from build123d import *

# Parameters (mm, degrees)
F0_R      = 1.75
F1_DEPTH  = 4
F3_W      = 3
F3_H      = 79.3
F4_DEPTH  = 82
F5_DEPTH  = 2
F6_DEPTH  = 2
F7_DEPTH  = 3
F8_DEPTH  = 3
F9_R      = 2
F12_DEPTH = 80.001
F14_W     = 58
F14_H     = 79.3
F14_W_2   = 22
F14_H_2   = 11
F15_DEPTH = 4


with BuildPart() as f1:
    # F0 (on Top) → F1 (new body)
    with BuildSketch(Plane.XY):
        Polygon((71, 89.45), (19, 89.45), (-6, 89.45), (-6, 81.45), (19, 81.45), (19, 15.45), (-6, 15.45), (-6, 7.45), (19, 7.45), (71, 7.45), (96, 7.45), (96, 15.45), (71, 15.45), (71, 81.45), (96, 81.45), (96, 89.45), align=None)
        with Locations((6.5, 11.45)):
            Circle(F0_R, mode=Mode.SUBTRACT)
        with Locations((83.5, 11.45)):
            Circle(F0_R, mode=Mode.SUBTRACT)
        with Locations((6.5, 85.45)):
            Circle(F0_R, mode=Mode.SUBTRACT)
        with Locations((83.5, 85.45)):
            Circle(F0_R, mode=Mode.SUBTRACT)
    extrude(amount=F1_DEPTH)

    # F3 (on offset) → F4 (join)
    with BuildSketch(Plane.XY.offset(4)):
        with Locations((20.5, 47.1)):
            Rectangle(F3_W, F3_H)
        with Locations((69.5, 47.1)):
            Rectangle(F3_W, F3_H)
    extrude(amount=F4_DEPTH)

    # F5 (cut): a face of the model
    f5_faces = [f1.faces().sort_by_distance(p)[0] for p in [
        (22, 47.1, 45),
    ]]
    extrude(f5_faces, amount=-F5_DEPTH, mode=Mode.SUBTRACT)

    # F6 (cut): a face of the model
    f6_faces = [f1.faces().sort_by_distance(p)[0] for p in [
        (68, 47.1, 45),
    ]]
    extrude(f6_faces, amount=-F6_DEPTH, mode=Mode.SUBTRACT)

    # F7 (add): a face of the model
    f7_faces = [f1.faces().sort_by_distance(p)[0] for p in [
        (71, 47.1526704697, 43.3223480034),
    ]]
    extrude(f7_faces, amount=F7_DEPTH)

    # F8 (add): a face of the model
    f8_faces = [f1.faces().sort_by_distance(p)[0] for p in [
        (19, 47.1526704697, 43.3223480034),
    ]]
    extrude(f8_faces, amount=F8_DEPTH)

    # F9
    f9_edges = [f1.edges().sort_by_distance(p)[0] for p in [
        (96, 81.45, 2),
        (96, 89.45, 2),
        (96, 15.45, 2),
        (96, 7.45, 2),
        (-6, 7.45, 2),
        (-6, 89.45, 2),
        (-6, 81.45, 2),
        (-6, 15.45, 2),
    ]]
    fillet(f9_edges, radius=F9_R)

    # F11 (on offset) → F12 (cut, through all)
    with BuildSketch(Plane.YZ.offset(74)):
        Polygon((73.4880973649, 79.5), (20.7553358046, 79.5), (17.45, 77.2472782643), (17.45, 6.3772784262), (20.6669158031, 4), (73.4427470628, 4), (76.75, 6.2499062224), (76.75, 77.1848345202), align=None)
    extrude(amount=-F12_DEPTH, mode=Mode.SUBTRACT)

    # F14 (on offset) → F15 (join)
    with BuildSketch(Plane.XY.offset(86)):
        with Locations((45, 47.1)):
            Rectangle(F14_W, F14_H)
        with Locations((55, 32.0759117305)):
            Rectangle(F14_W_2, F14_H_2, mode=Mode.SUBTRACT)
    extrude(amount=F15_DEPTH)


solid = f1.part
The model under review builds one solid part; all positions refer to its coordinate system, in mm. A direction names the side the tool comes from. Round coordinates to 2 decimals unless told otherwise and drop trailing zeros. Loops run counter-clockwise (first coordinate to the right, second up) from the corner with the lowest first, then second, coordinate; pieces in that order, holes last. Notation, with made-up numbers: M 43,79.5 L 83,79.5 A16 cw 83,106.5 Z; hole C -21.75,49.25 d4. An arc over 180 degrees is marked long. Answer as a JSON object with one key per item and string values.
Item 1: We need section C-C, the plane x = 83.5. State the section outline as (y, z) points, and give its area (3 significant figures).
Check sheet entries:
{"outline": "M 7.45,0 L 9.7,0 L 9.7,4 L 7.45,4 Z; M 13.2,0 L 15.45,0 L 15.45,4 L 13.2,4 Z; M 81.45,0 L 83.7,0 L 83.7,4 L 81.45,4 Z; M 87.2,0 L 89.45,0 L 89.45,4 L 87.2,4 Z", "area": "36.0 mm2"}
Item 2: We need section B-B, the plane z = 59. State the section outline as (x, y) points.
Check sheet entries:
{"outline": "M 16,7.45 L 20,7.45 L 20,17.45 L 16,17.45 Z; M 16,76.75 L 20,76.75 L 20,86.75 L 16,86.75 Z; M 70,7.45 L 74,7.45 L 74,17.45 L 70,17.45 Z; M 70,76.75 L 74,76.75 L 74,86.75 L 70,86.75 Z"}
Item 3: We need section A-A, the plane y = 11.45. State the section outline as (x, z) points.
Check sheet entries:
{"outline": "M -6,0 L 4.75,0 L 4.75,4 L -6,4 Z; M 8.25,0 L 81.75,0 L 81.75,4 L 74,4 L 74,90 L 16,90 L 16,4 L 8.25,4 Z; M 85.25,0 L 96,0 L 96,4 L 85.25,4 Z; hole M 20,4 L 70,4 L 70,86 L 20,86 Z"}
Item 4: Tool access review of faces 1 (the face through (6, 15.45, 2)), 2 (the face through (84, 81.45, 2)), 3 (the face through (72.028, 75.142, 78.326)), 4 (the face through (4.8, 12.4, 4)): name each direction out of +Z, -Z, +X, -X, +Y, -Y from which nothing blocks a thin tool from reaching the whole face with its end or side.
Check sheet entries:
{"face 1": "+Z, -Z, -X", "face 2": "+Z, -Z, +X", "face 3": "+X, -X", "face 4": "+Z, -X, +Y, -Y"}
Item 5: The part is to be moulded in two halves that separate along X. For faces 5 (the face through (72, 76.75, 41)), 6 (the face through (84.31, 83.9, 1.97)), say which applies: +X half, -X half, draft (parallel to the pull), parting line (faces both ways), or undercut.
Check sheet entries:
{"face 5": "draft", "face 6": "undercut"}
Item 6: Clearance check with flat-ended pins moving along their axes: P1, Ø10, axis at x = 25.5, y = 30.5, coming from the -Z side; P2, Ø3, axis at x = 6.5, y = 11.45, coming from the +Z side; P3, Ø3, axis at x = 60, z = 88, coming from the +Y side; P4, Ø3, axis at y = 34, z = 89, coming from the -X side. State where each tip first meets the part, or that it passes through.
Check sheet entries:
{"P1": "z = 0", "P2": "through", "P3": "y = 86.75", "P4": "x = 16"}
Item 7: We need section D-D, the plane y = 54.5. State the section outline as (x, z) points, and give its area (3 significant figures).
Check sheet entries:
{"outline": "M 16,0 L 74,0 L 74,4 L 16,4 Z; M 16,79.5 L 20,79.5 L 20,86 L 70,86 L 70,79.5 L 74,79.5 L 74,90 L 16,90 Z", "area": "516 mm2"}
Item 8: For line 1 along Y through (x, z) = (83.5, 2.5); line 2 along X through (y, z) = (85.45, 2.15); line 3 along Z through (x, y) = (41, 32.5), list the stretches that pass through material, from the lowest coordinate up.
Check sheet entries:
{"line 1": "7.45 to 9.7, 13.2 to 15.45, 81.45 to 83.7, 87.2 to 89.45", "line 2": "-6 to 4.75, 8.25 to 81.75, 85.25 to 96", "line 3": "0 to 4, 86 to 90"}
